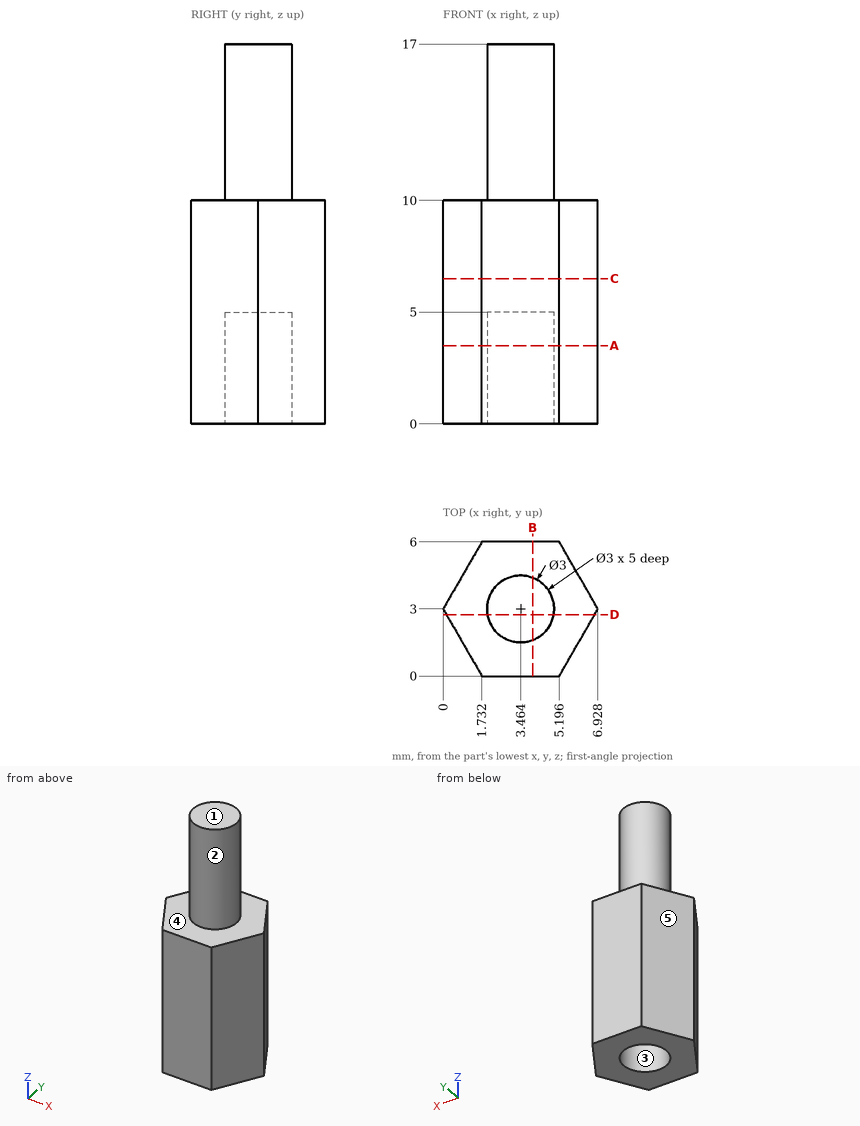
Geometry check sheet. Reference: drawing and pictorial views, mm from the part's lowest x, y, z. A direction names the side the tool comes from. Give positions to 0.01 mm unless a question says otherwise; leave off trailing zeros. Order: outer loops, then holes, each group sorted by start corner. A loop starts at its lowest first (then second) coordinate and runs counter-clockwise, first axis right, second up. Notation, with made-up numbers: M 80,9 L 117,9 A22 cw 117,18 Z; hole C 1.5,45 d7. An arc over 180 degrees is marked long. Return JSON: item names as keys, results as strings. Group by question number.
1) Section check A-A on z = 3.5. Record the cut outline in (x, y).
2) Section check B-B on x = 4. Record the cut outline in (y, z), and give its area (3 significant figures).
3) Section check C-C on z = 6.5. Record the cut outline in (x, y).
4) Scan lines: line 1 (Z direction, x = 5.75, y = 1.5); line 2 (Z direction, x = 3.5, y = 3.75); line 3 (Y direction, x = 2.75, z = 1.25). Record each from-to range of solid material in increasing order.
5) Access from +Z, -Z, +X, -X, +Y, -Y to the whole of each face (thin tool, end or side, straight path). Record for the marked faces 1 and 2.
6) Mould release check, pull along X, two halves, no side actions. Record for the marked faces 3, 4 and 5: pulls with the +X half, pulls with the -X half, needs draft (parallel to the pull), parting line crosses it, or undercut.
7) Section check D-D on y = 2.75. Record the cut outline in (x, z) (1 decimal).
8) Go/stop test with a flat-tipped pin: pin 1 Ø2 at (x, y) = (4.5, 5) entering from -Z. Record where the tip stops, or that it passes through.
Answer block:
{
 "1": {"outline": "M 0,3 L 1.73,0 L 5.2,0 L 6.93,3 L 5.2,6 L 1.73,6 Z; hole C 3.46,3 d3"},
 "2": {"outline": "M 0,0 L 1.6,0 L 1.6,5 L 4.4,5 L 4.4,0 L 6,0 L 6,10 L 4.4,10 L 4.4,17 L 1.6,17 L 1.6,10 L 0,10 Z", "area": "65.6 mm^2"},
 "3": {"outline": "M 0,3 L 1.73,0 L 5.2,0 L 6.93,3 L 5.2,6 L 1.73,6 Z"},
 "4": {"line 1": "z = 0 to 10", "line 2": "z = 5 to 17", "line 3": "y = 0 to 1.68, 4.32 to 6"},
 "5": {"face 1": "+Z, +X, -X, +Y, -Y", "face 2": "+Z"},
 "6": {"face 3": "undercut", "face 4": "needs draft", "face 5": "pulls with the -X half"},
 "7": {"outline": "M 0.1,0 L 2,0 L 2,5 L 4.9,5 L 4.9,0 L 6.8,0 L 6.8,10 L 4.9,10 L 4.9,17 L 2,17 L 2,10 L 0.1,10 Z"},
 "8": {"pin 1": "stops at z = 0"}
}
